Source: CAD feature listing. Evaluate the final solid. Frame: model axes, mm. Face numbers are marked on the shaded views. A direction names the side the tool comes from. Round coordinates to 2 decimals unless told otherwise and drop trailing zeros. Write each loop counter-clockwise with the first axis right and the second up, starting at its lowest first coordinate (ties: lowest second). Pieces come first, ordered by that corner, then holes. Notation, with made-up numbers: M -36.5,64.5 L -23.5,64.5 A32 ccw -23.5,96.5 Z; hole C -6.5,23 d10. An arc over 180 degrees is marked long. Answer in a Markdown table with one row per item. Add a question column.
Item 1: Cut plane C-C on z = -52.57. Return loops of the section in (x, y), and give its area (3 significant figures).
Item 2: Material intervals for probe 1 along Y at (x, z) = (60.5, 3.35); probe 2 along X at (y, z) = (61.6, -52.57); probe 3 along Z at (x, y) = (43, 26.5), sorted ascending.
Item 3: Mould query, pull axis Z, two halves, no side actions, for the marked faces 1, 2 and 3. Classes: released by +Z, released by -Z, zero draft, split by the parting line, or undercut.
Item 4: Contact query for flat-ended pins moving along their axis: pin 1 (12 mm diameter, centred on x = 48, z = -10.5, fed in from -Y); pin 2 (4 mm diameter, centred on y = 42.955, z = -3.695, fed in from +X); pin 3 (2 mm diameter, centred on x = 7, z = -45.5, fed in from +Y); pin 4 (7 mm diameter, centred on x = 1.5, y = 19, fed in from -Z). Output: stop coordinate, or through.
Item 5: Set-up query: the marked faces 4, 5, 6 and 7. Return all of +Z, -Z, +X, -X, +Y, -Y with unobstructed straight access to the full face (end or side cutting, diameter ignored); none if empty.
Item 6: Cut plane A-A on z = -21.66. Return loops of the section in (x, y).
Item 7: Cut plane B-B on y = 25. Return loops of the section in (x, z).
Item 8: Cut plane D-D on x = 4.5. Return loops of the section in (y, z) (3 decimals).
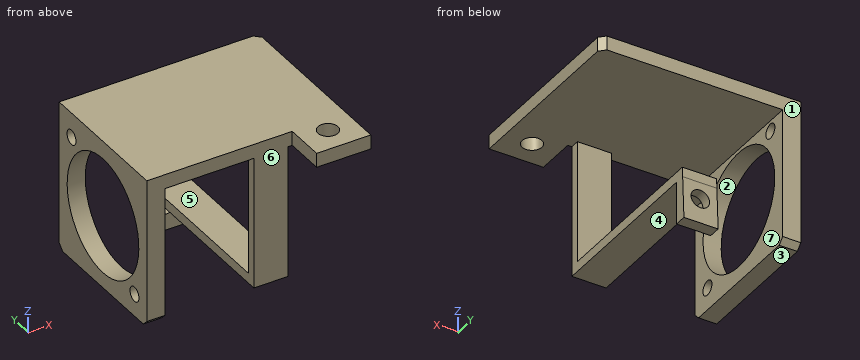
from build123d import *

# Parameters (mm, degrees)
BOSS_EXTRUDE1_DEPTH  = 5
SKETCH2_W            = 6.35
SKETCH2_H            = 50
BOSS_EXTRUDE2_DEPTH  = 52.48
CUT_EXTRUDE1_REACH   = 106.448
SKETCH3_R            = 20.44
SKETCH3_R_2          = 2.555
SKETCH3_W            = 5
SKETCH3_H            = 50
CUT_EXTRUDE2_REACH   = 108.104
SKETCH4_R            = 3.5
CUT_EXTRUDE6_REACH   = 108.104
SKETCH14_W           = 23.196263878
SKETCH14_H           = 15.316152196
SKETCH15_W           = 12
SKETCH15_H           = 3.2
BOSS_EXTRUDE7_DEPTH  = 46.5
BOSS_EXTRUDE8_REACH  = 98.667
SKETCH16_W           = 12
SKETCH16_H           = 3.5
SKETCH17_W           = 12
SKETCH17_H           = 3.5
BOSS_EXTRUDE9_DEPTH  = 15
CHAMFER2_SIZE        = 2
SKETCH22_W           = 12
SKETCH22_H           = 15
BOSS_EXTRUDE10_DEPTH = 0.72
CUT_EXTRUDE8_REACH   = 103.606
CUT_EXTRUDE7_REACH   = 120.762
SKETCH18_R           = 3.25


with BuildPart() as part:
    # Sketch1 → Boss-Extrude1 (new body)
    with BuildSketch(Plane.XY):
        Polygon((0, 0), (0, 50), (51, 50), (51, 64.061014889), (70, 64.061014889), (70, -13.938985111), (51, -13.938985111), (51, 0), align=None)
    extrude(amount=BOSS_EXTRUDE1_DEPTH)

    # Sketch2 → Boss-Extrude2 (add)
    with BuildSketch(Plane(origin=(0, 0, 0), x_dir=(-1, 0, 0), z_dir=(0, 0, -1))):
        with Locations((-3.175, 25)):
            Rectangle(SKETCH2_W, SKETCH2_H)
    extrude(amount=BOSS_EXTRUDE2_DEPTH)

    # Sketch3 → Cut-Extrude1 (cut, up to next)
    with BuildSketch(Plane(origin=(6.35, 0, 0), x_dir=(0, 0, -1), z_dir=(1, 0, 0)), mode=Mode.PRIVATE) as cut_extrude1_sk1:
        with Locations((21.66, 25)):
            Circle(SKETCH3_R)
    cut_extrude1_tool1 = extrude(cut_extrude1_sk1.sketch, amount=-CUT_EXTRUDE1_REACH, mode=Mode.PRIVATE) & part.part
    # Sketch3 → Cut-Extrude1 (cut, up to next)
    with BuildSketch(Plane(origin=(6.35, 0, 0), x_dir=(0, 0, -1), z_dir=(1, 0, 0)), mode=Mode.PRIVATE) as cut_extrude1_sk2:
        with Locations((3.695, 42.955)):
            Circle(SKETCH3_R_2)
    cut_extrude1_tool2 = extrude(cut_extrude1_sk2.sketch, amount=-CUT_EXTRUDE1_REACH, mode=Mode.PRIVATE) & part.part
    # Sketch3 → Cut-Extrude1 (cut, up to next)
    with BuildSketch(Plane(origin=(6.35, 0, 0), x_dir=(0, 0, -1), z_dir=(1, 0, 0)), mode=Mode.PRIVATE) as cut_extrude1_sk3:
        with Locations((39.615, 7.045)):
            Circle(SKETCH3_R_2)
    cut_extrude1_tool3 = extrude(cut_extrude1_sk3.sketch, amount=-CUT_EXTRUDE1_REACH, mode=Mode.PRIVATE) & part.part
    # Sketch3 → Cut-Extrude1 (cut, up to next)
    with BuildSketch(Plane(origin=(6.35, 0, 0), x_dir=(0, 0, -1), z_dir=(1, 0, 0)), mode=Mode.PRIVATE) as cut_extrude1_sk4:
        with Locations((49.98, 25)):
            Rectangle(SKETCH3_W, SKETCH3_H)
    cut_extrude1_tool4 = extrude(cut_extrude1_sk4.sketch, amount=-CUT_EXTRUDE1_REACH, mode=Mode.PRIVATE) & part.part
    add(cut_extrude1_tool1.solids().sort_by_distance((6.35, 25, -21.66))[0], mode=Mode.SUBTRACT)
    add(cut_extrude1_tool2.solids().sort_by_distance((6.35, 42.955, -3.695))[0], mode=Mode.SUBTRACT)
    add(cut_extrude1_tool3.solids().sort_by_distance((6.35, 7.045, -39.615))[0], mode=Mode.SUBTRACT)
    add(cut_extrude1_tool4.solids().sort_by_distance((6.35, 25, -49.98))[0], mode=Mode.SUBTRACT)

    # Sketch4 → Cut-Extrude2 (cut, up to next)
    with BuildSketch(Plane(origin=(0, 0, 0), x_dir=(-1, 0, 0), z_dir=(0, 0, -1)), mode=Mode.PRIVATE) as cut_extrude2_sk1:
        with Locations((-60.5, 55.061014889)):
            Circle(SKETCH4_R)
    cut_extrude2_tool1 = extrude(cut_extrude2_sk1.sketch, amount=-CUT_EXTRUDE2_REACH, mode=Mode.PRIVATE) & part.part
    # Sketch4 → Cut-Extrude2 (cut, up to next)
    with BuildSketch(Plane(origin=(0, 0, 0), x_dir=(-1, 0, 0), z_dir=(0, 0, -1)), mode=Mode.PRIVATE) as cut_extrude2_sk2:
        with Locations((-60.5, -4.938985111)):
            Circle(SKETCH4_R)
    cut_extrude2_tool2 = extrude(cut_extrude2_sk2.sketch, amount=-CUT_EXTRUDE2_REACH, mode=Mode.PRIVATE) & part.part
    add(cut_extrude2_tool1.solids().sort_by_distance((60.5, 55.061015, 0))[0], mode=Mode.SUBTRACT)
    add(cut_extrude2_tool2.solids().sort_by_distance((60.5, -4.938985, 0))[0], mode=Mode.SUBTRACT)

    # Sketch14 → Cut-Extrude6 (cut, up to next)
    with BuildSketch(Plane(origin=(0, 0, 0), x_dir=(-1, 0, 0), z_dir=(0, 0, -1)), mode=Mode.PRIVATE) as cut_extrude6_sk1:
        with Locations((-62.598131939, 57.658076098)):
            Rectangle(SKETCH14_W, SKETCH14_H)
    cut_extrude6_tool1 = extrude(cut_extrude6_sk1.sketch, amount=-CUT_EXTRUDE6_REACH, mode=Mode.PRIVATE) & part.part
    add(cut_extrude6_tool1.solids().sort_by_distance((62.598132, 57.658076, 0))[0], mode=Mode.SUBTRACT)

    # Sketch15 → Boss-Extrude7 (add)
    with BuildSketch(Plane(origin=(0, 0, 0), x_dir=(-1, 0, 0), z_dir=(0, 0, -1))):
        with Locations((-43.56, 1.6)):
            Rectangle(SKETCH15_W, SKETCH15_H)
    extrude(amount=BOSS_EXTRUDE7_DEPTH)

    # Boss-Extrude8: up to this plane
    boss_extrude8_end = Plane(origin=(166.832994776, 64.085435133, -66.619565524), z_dir=(-1.1416993347548052e-15, 0.9990256874715413, 0.04413247978546202))
    # Sketch16 → Boss-Extrude8 (add, up to the surface)
    with BuildSketch(Plane(origin=(0, 3.2, 0), x_dir=(1, 0, 0), z_dir=(0, 1, 0)), mode=Mode.PRIVATE) as boss_extrude8_sk1:
        with Locations((43.56, 44.75)):
            Rectangle(SKETCH16_W, SKETCH16_H)
    boss_extrude8_tool1 = split(extrude(boss_extrude8_sk1.sketch, amount=BOSS_EXTRUDE8_REACH, mode=Mode.PRIVATE), bisect_by=boss_extrude8_end, keep=Keep.BOTH, mode=Mode.PRIVATE)
    add(boss_extrude8_tool1.solids().sort_by_distance((43.56, 3.2, -44.75))[0])

    # Sketch17 → Boss-Extrude9 (add)
    with BuildSketch(Plane(origin=(0, 0, -46.5), x_dir=(-1, 0, 0), z_dir=(0, 0, -1))):
        with Locations((-43.56, 61.446642853)):
            Rectangle(SKETCH17_W, SKETCH17_H)
    extrude(amount=BOSS_EXTRUDE9_DEPTH)

    # Chamfer2
    chamfer2_edges = [part.edges().sort_by_distance(p)[0] for p in [
        (3.175, 0, -47.48),
        (3.175, 50, -47.48),
        (70, 50, 2.5),
    ]]
    chamfer(chamfer2_edges, length=CHAMFER2_SIZE)

    # Sketch22 → Boss-Extrude10 (add)
    with BuildSketch(Plane(origin=(0, 63.196642853, 0), x_dir=(1, 0, 0), z_dir=(0, 1, 0))):
        with Locations((43.56, 54)):
            Rectangle(SKETCH22_W, SKETCH22_H)
    extrude(amount=BOSS_EXTRUDE10_DEPTH)

    # Sketch23 → Cut-Extrude8 (cut, up to next)
    with BuildSketch(Plane(origin=(49.56, 0, 0), x_dir=(0, 0, -1), z_dir=(1, 0, 0)), mode=Mode.PRIVATE) as cut_extrude8_sk1:
        Polygon((46.5, 63.916642853), (46.5, 63.196642853), (61.5, 63.916642853), align=None)
    cut_extrude8_tool1 = extrude(cut_extrude8_sk1.sketch, amount=-CUT_EXTRUDE8_REACH, mode=Mode.PRIVATE) & part.part
    add(cut_extrude8_tool1.solids().sort_by_distance((49.56, 63.676643, -51.5))[0], mode=Mode.SUBTRACT)

    # Cut-Extrude7: up to this plane
    cut_extrude7_end = Plane(origin=(-0.001, 63.196642853, -46.5), z_dir=(-2.1659106514416256e-15, -0.9988499868416298, -0.04794479936839813))
    # Sketch18 → Cut-Extrude7 (cut, up to the surface)
    with BuildSketch(Plane.XZ.offset(-59.696642853), mode=Mode.PRIVATE) as cut_extrude7_sk1:
        with Locations(Location((43.56, -52.57, 0), (0, 0, 270))):
            Circle(SKETCH18_R)
    cut_extrude7_tool1 = split(extrude(cut_extrude7_sk1.sketch, amount=-CUT_EXTRUDE7_REACH, mode=Mode.PRIVATE), bisect_by=cut_extrude7_end, keep=Keep.BOTH, mode=Mode.PRIVATE)
    add(cut_extrude7_tool1.solids().sort_by_distance((43.56, 59.696643, -52.57))[0], mode=Mode.SUBTRACT)


solid = part.part
Results below:
| question | item | result |
|---|---|---|
| 1 | outline | M 37.56,59.7 L 40.31,59.7 L 40.31,63.49 L 37.56,63.49 Z; M 46.81,59.7 L 49.56,59.7 L 49.56,63.49 L 46.81,63.49 Z |
| 1 | area | 20.9 mm2 |
| 2 | probe 1 | -13.94 to -8.44, -1.44 to 50 |
| 2 | probe 2 | 37.56 to 40.31, 46.81 to 49.56 |
| 2 | probe 3 | -46.5 to -43, 0 to 5 |
| 3 | face 1 | zero draft |
| 3 | face 2 | undercut |
| 3 | face 3 | released by -Z |
| 4 | pin 1 | y = 0 |
| 4 | pin 2 | through |
| 4 | pin 3 | y = 50 |
| 4 | pin 4 | z = -47.48 |
| 5 | face 4 | -Z, +X, -Y |
| 5 | face 5 | +X, +Y |
| 5 | face 6 | +Z, -Z, -X, -Y |
| 5 | face 7 | -Z, +Y, -Y |
| 6 | outline | M 0,0 L 6.35,0 L 6.35,4.56 L 0,4.56 Z; M 0,45.44 L 6.35,45.44 L 6.35,50 L 0,50 Z; M 37.56,0 L 49.56,0 L 49.56,3.2 L 37.56,3.2 Z |
| 7 | outline | M 0,-47.48 L 6.35,-47.48 L 6.35,-42.1 L 0,-42.1 Z; M 0,-1.22 L 6.35,-1.22 L 6.35,0 L 70,0 L 70,5 L 0,5 Z; M 37.56,-46.5 L 49.56,-46.5 L 49.56,-43 L 37.56,-43 Z |
| 8 | outline | M 0,-45.48 L 2,-47.48 L 48,-47.48 L 50,-45.48 L 50,5 L 0,5 Z; hole C 7.045,-39.615 d5.11; hole C 25,-21.66 d40.88; hole C 42.955,-3.695 d5.11 |
